from build123d import *

# Parameters (mm, degrees)
EXTRUDE1_DEPTH = 21
SKETCH3_R      = 1.5875
EXTRUDE2_DEPTH = 3
SKETCH4_R      = 3.15
EXTRUDE3_DEPTH = 3


with BuildPart() as part:
    # Sketch2 → Extrude1 (new body)
    with BuildSketch(Plane(origin=(0, 0, 0), x_dir=(0, 0, -1), z_dir=(1, 0, 0))):
        with BuildLine():
            Line((0, 4), (0, 21))
            Line((0, 21), (-3, 21))
            Line((-3, 21), (-3, 4))
            ThreePointArc((-3, 4), (-3.292893219, 3.292893219), (-4, 3))
            Line((-4, 3), (-22.5, 3))
            Line((-22.5, 3), (-22.5, 0))
            Line((-22.5, 0), (-4, 0))
            ThreePointArc((-4, 0), (-1.171572875, 1.171572875), (0, 4))
        make_face()
    extrude(amount=EXTRUDE1_DEPTH)

    # Sketch3 → Extrude2 (cut)
    with BuildSketch(Plane(origin=(0, 3, 0), x_dir=(1, 0, 0), z_dir=(0, 1, 0))):
        with Locations(Location((10.5, -13.8, 0), (0, 0, 270))):
            Circle(SKETCH3_R)
    extrude(amount=-EXTRUDE2_DEPTH, mode=Mode.SUBTRACT)

    # Sketch4 → Extrude3 (cut)
    with BuildSketch(Plane.XY.offset(3)):
        with Locations((10.5, 13.8)):
            Circle(SKETCH4_R)
    extrude(amount=-EXTRUDE3_DEPTH, mode=Mode.SUBTRACT)


solid = part.part
Design review of the part built by this model. Coordinates are the model's own, in mm. A direction names the side the tool comes from. Round coordinates to 2 decimals unless told otherwise and drop trailing zeros. Loops run counter-clockwise (first coordinate to the right, second up) from the corner with the lowest first, then second, coordinate; pieces in that order, holes last. Notation, with made-up numbers: M 32.25,1 L 67.25,1 A27 ccw 67.25,28 Z; hole C 5.5,20.25 d2. An arc over 180 degrees is marked long. Answer as a JSON object with one key per item and string values.
Item 1: Wall thickness on L1, parallel to X at y = 2.1, z = 13.8; L2, parallel to Z at x = 19.75, y = 5: over which ranges is each line inside the solid? List them lowest first. Write a range as from..to.
Answer sheet:
{"L1": "x = 0..8.91, 12.09..21", "L2": "z = 0..3"}
Item 2: The part is to be moulded in two halves that separate along Z. For faces 1 (the flat face through (10, 10, 0)), 2 (the cylindrical face through (10.353, 3.301, 3.285)), 3 (the flat face through (21, 2.8, 8)), 4 (the cylindrical face through (9.892, 1.521, 15.266)), say which applies: pulls with the +Z half, pulls with the -Z half, needs draft (parallel to the pull), parting line crosses it, or undercut.
Answer sheet:
{"face 1": "pulls with the -Z half", "face 2": "pulls with the +Z half", "face 3": "needs draft", "face 4": "undercut"}
Item 3: We need section D-D on x = 6.5. Give the boundary of the cut face in (y, z), and give its area (3 significant figures).
Answer sheet:
{"outline": "M 0,4 A4 ccw 4,0 L 21,0 L 21,3 L 4,3 A1 cw 3,4 L 3,22.5 L 0,22.5 Z", "area": "118 mm^2"}
Item 4: We need section A-A on x = 10.5. Give the boundary of the cut face in (y, z), and give its area (3 significant figures).
Answer sheet:
{"outline": "M 0,4 A4 ccw 4,0 L 10.65,0 L 10.65,3 L 4,3 A1 cw 3,4 L 3,12.21 L 0,12.21 Z; M 0,15.39 L 3,15.39 L 3,22.5 L 0,22.5 Z; M 16.95,0 L 21,0 L 21,3 L 16.95,3 Z", "area": "89.9 mm^2"}
Item 5: Clearance check with flat-ended pins moving along their axes: P1, Ø2, axis at y = 5, z = 5, coming from the +X side; P2, Ø8, axis at x = 6.5, y = 17, coming from the -Z side; P3, Ø3.5, axis at x = 10.5, z = 13.8, coming from the +Y side; P4, Ø4, axis at x = 17.5, y = 6, coming from the +Z side. State where each tip first meets the part, or that it passes through.
Answer sheet:
{"P1": "passes through", "P2": "stops at z = 0", "P3": "stops at y = 3", "P4": "stops at z = 3"}
Item 6: Machinability: for faces 5 (the flat face through (10, 2, 22.5)), 6 (the flat face through (10, 3, 11)), which of the approach directions +Z, -Z, +X, -X, +Y, -Y give a long, thin tool a straight path to every point of the face, cutting with its end or side? Answer none if there is none.
Answer sheet:
{"face 5": "+Z, +X, -X, +Y, -Y", "face 6": "+Z, +X, -X, +Y"}
Item 7: We need section C-C on z = 13.75. Give the boundary of the cut face in (x, y), and give its area (3 significant figures).
Answer sheet:
{"outline": "M 0,0 L 8.91,0 L 8.91,3 L 0,3 Z; M 12.09,0 L 21,0 L 21,3 L 12.09,3 Z", "area": "53.5 mm^2"}
Item 8: We need section B-B on y = 13.8. Give the boundary of the cut face in (x, z), and give its area (3 significant figures).
Answer sheet:
{"outline": "M 0,0 L 7.35,0 L 7.35,3 L 0,3 Z; M 13.65,0 L 21,0 L 21,3 L 13.65,3 Z", "area": "44.1 mm^2"}
